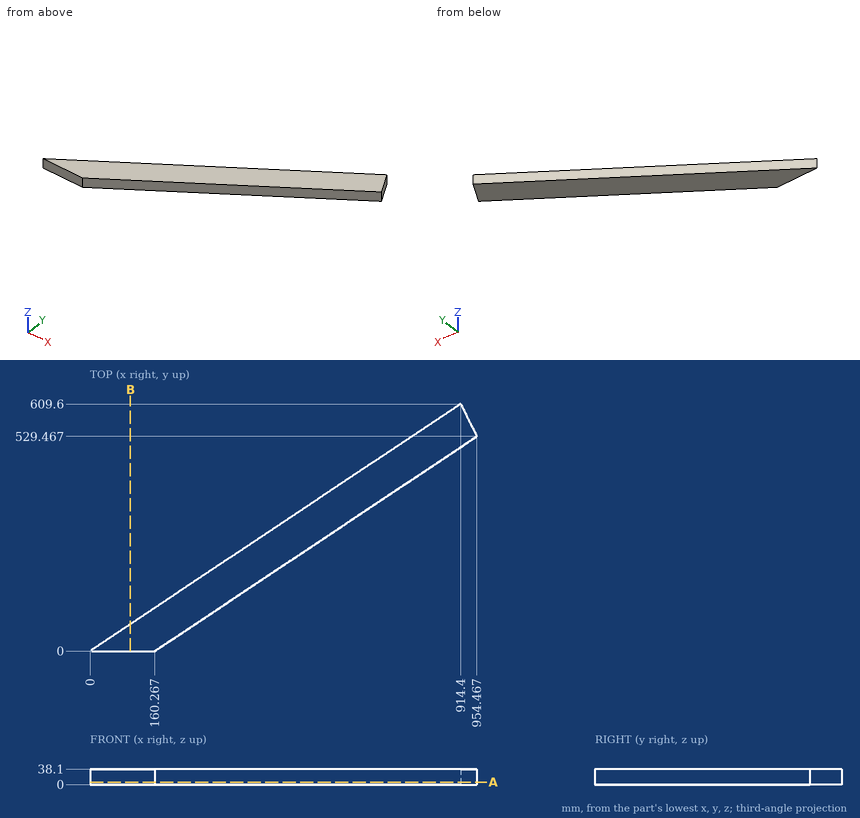
Input: dimensioned drawing with shaded views. Units: mm. Origin: part minimum x, y, z. Give positions to 0.01 mm unless a question says otherwise; leave off trailing zeros. Write each loop counter-clockwise with the first axis right and the second up, starting at its lowest first coordinate (ties: lowest second). Pieces come first, ordered by that corner, then holes.
1. Section query A-A (z = 6). Return the cut outline in (x, y).
2. Section query B-B (x = 99.5). Return the cut outline in (y, z), then the cut area to 3 significant figures.
3. Material intervals for line 1 along Y through (x, z) = (377, 33) (1 decimal); line 2 along Y through (x, z) = (228, 19) (1 decimal); line 3 along X through (y, z) = (96, 21) (1 decimal), sorted ascending.
4. First-contact query: pin 1 (5 mm diameter, centred on y = 172, z = 24, fed in from +X) (1 decimal); pin 2 (2 mm diameter, centred on y = 464.5, z = 20.5, fed in from +X) (1 decimal); pin 3 (1 mm diameter, centred on x = 726.5, z = 22, fed in from -Y) (1 decimal). Flat tips, straight axial feed; report the tip coordinate or a pass-through.
Output values:
1. outline: (0, 0) - (160.27, 0) - (954.47, 529.47) - (914.4, 609.6) - close
2. outline: (0, 0) - (66.33, 0) - (66.33, 38.1) - (0, 38.1) - close
2. area: 2,530 mm2
3. line 1: y = 144.5 to 251.3
3. line 2: y = 45.2 to 152
3. line 3: x = 144 to 304.3
4. pin 1: stops at x = 422
4. pin 2: stops at x = 858.5
4. pin 3: stops at y = 377.2
